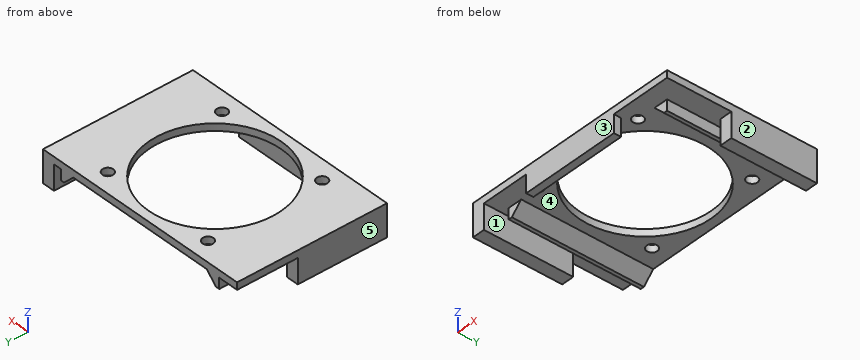
from build123d import *

# Parameters (mm, degrees)
SKETCH_1_W      = 62
SKETCH_1_H      = 42
SKETCH_1_R      = 18.5
EXTRUDE_1_DEPTH = 2
F_3_0MM_1_D     = 3
SKETCH_4_W      = 3.5
SKETCH_4_H      = 24
SKETCH_4_H_2    = 25
EXTRUDE_2_DEPTH = 7
SKETCH_5_W      = 28
SKETCH_5_H      = 2
EXTRUDE_3_DEPTH = 5
SKETCH_7_W      = 4
SKETCH_7_H      = 37
EXTRUDE_4_DEPTH = 3
CHAMFER_1_SIZE  = 3


with BuildPart() as part:
    # 스케치1 → 보스-돌출1 (new body)
    with BuildSketch(Plane.XY):
        Rectangle(SKETCH_1_W, SKETCH_1_H)
        Circle(SKETCH_1_R, mode=Mode.SUBTRACT)
    extrude(amount=EXTRUDE_1_DEPTH)

    # Ø3.0mm 맞춤핀 구멍1 (through all)
    with Locations(Plane(origin=(-16, 16, 2), x_dir=(1, 0, 0), z_dir=(0, 0, 1))):
        with Locations((0, 0), (32, 0), (32, -32), (0, -32)):
            Hole(F_3_0MM_1_D / 2)

    # 스케치4 → 보스-돌출2 (add)
    with BuildSketch(Plane(origin=(0, 0, 0), x_dir=(-1, 0, 0), z_dir=(0, 0, -1))):
        with Locations((-29.25, 9)):
            Rectangle(SKETCH_4_W, SKETCH_4_H)
        with Locations((29.25, -8.5)):
            Rectangle(SKETCH_4_W, SKETCH_4_H_2)
    extrude(amount=EXTRUDE_2_DEPTH)

    # 스케치5 → 보스-돌출3 (add)
    with BuildSketch(Plane(origin=(0, 0, 0), x_dir=(-1, 0, 0), z_dir=(0, 0, -1))):
        with Locations((0, -20)):
            Rectangle(SKETCH_5_W, SKETCH_5_H)
    extrude(amount=EXTRUDE_3_DEPTH)

    # 스케치7 → 보스-돌출4 (add)
    with BuildSketch(Plane(origin=(0, 0, 0), x_dir=(-1, 0, 0), z_dir=(0, 0, -1))):
        with Locations((-23.3, 2.5)):
            Rectangle(SKETCH_7_W, SKETCH_7_H)
        with Locations((23.3, 2.5)):
            Rectangle(SKETCH_7_W, SKETCH_7_H)
    extrude(amount=EXTRUDE_4_DEPTH)

    # 모따기1
    chamfer_1_edges = [part.edges().sort_by_distance(p)[0] for p in [
        (-21.3, 2.5, -3),
        (21.3, 2.5, -3),
    ]]
    chamfer(chamfer_1_edges, length=CHAMFER_1_SIZE - 0.0001)  # a hair under: the kernel refuses the full size


solid = part.part
Work out the finished part from the listing and answer in its coordinate system (mm). Face numbers are marked on the shaded views. A direction names the side the tool comes from. Coordinates: 2 decimals unless noted, no trailing zeros. Loops run counter-clockwise (first coordinate to the right, second up) from the corner with the lowest first, then second, coordinate; pieces in that order, holes last. Notation, with made-up numbers: (25.25, -0.75) -> (82.25, -0.75) arc R37 ccw to (82.25, 36.25) -> close; hole circle Ø11 at (-38, -12.5). An arc over 180 degrees is marked (long way). Answer as CSV lines item,"result".
1) For a pull along X with two mould halves and no side action, classify the marked faces 3, 4 and 5 as released by +X, released by -X, zero draft, split by the parting line, or undercut.
A:
face 3,"zero draft"
face 4,"undercut"
face 5,"released by -X"
2) Flat-ended cylindrical pins translate along their axes: pin 1 (0.8 mm diameter, centred on x = -25, y = 2, fed in from -Z); pin 2 (1 mm diameter, centred on y = -6.5, z = -3, fed in from +X); pin 3 (1.5 mm diameter, centred on x = -24.5, z = -1, fed in from -Y). Find the tip coordinate at first contact, or state that the pin passes through.
A:
pin 1,"stops at z = -3"
pin 2,"stops at x = 25.3"
pin 3,"stops at y = -16"
3) Straight lines are drawn through the part: probe 1 along X at (y, z) = (18.5, -2.5); probe 2 along X at (y, z) = (7, -2.75); probe 3 along Y at (x, z) = (0, 1.4). For each, find the intervals that lie inside material, in ascending order.
A:
probe 1,"x = -25.3 to -23.8, 23.8 to 25.3, 27.5 to 31"
probe 2,"x = -25.3 to -24.05, 24.05 to 25.3, 27.5 to 31"
probe 3,"y = -21 to -18.5, 18.5 to 21"
4) The part is cut by section D-D (x = 0). Give the vertices of the cut face in (y, z).
A:
outline,"(-21, -5) -> (-19, -5) -> (-19, 0) -> (-18.5, 0) -> (-18.5, 2) -> (-21, 2) -> close; (18.5, 0) -> (21, 0) -> (21, 2) -> (18.5, 2) -> close"
5) The part is cut by section C-C (y = 16). State how many separate pieces and enclosed holes the cut face has, and give its area (3 significant figures).
A:
separate pieces,"4"
enclosed holes,"0"
area,"114 mm²"
6) The part is cut by section A-A (z = 1). Give the vertices of the cut face in (x, y).
A:
outline,"(-31, -21) -> (31, -21) -> (31, 21) -> (-31, 21) -> close; hole circle Ø37 at (0, 0); hole circle Ø3 at (-16, -16); hole circle Ø3 at (-16, 16); hole circle Ø3 at (16, -16); hole circle Ø3 at (16, 16)"
7) For the marked faces 1 and 2, determine the directions among +Z, -Z, +X, -X, +Y, -Y from which every point of the face is accessible in a straight line to the end or side of a thin tool.
A:
face 1,"-Z, +Y, -Y"
face 2,"+Z, -Z, +X, +Y, -Y"
8) The part is cut by section B-B (z = -3.75). Give the vertices of the cut face in (x, y), and give its area (4 significant figures).
A:
outline,"(-31, -21) -> (-27.5, -21) -> (-27.5, 4) -> (-31, 4) -> close; (-14, -21) -> (14, -21) -> (14, -19) -> (-14, -19) -> close; (27.5, -3) -> (31, -3) -> (31, 21) -> (27.5, 21) -> close"
area,"227.5 mm²"
